Geometry check sheet. Reference: the model listing, model coordinates, mm. A direction names the side the tool comes from. Give positions to 0.01 mm unless a question says otherwise; leave off trailing zeros. Order: outer loops, then holes, each group sorted by start corner. A loop starts at its lowest first (then second) coordinate and runs counter-clockwise, first axis right, second up. Notation, with made-up numbers: M -8.75,83.25 L 16.25,83.25 A37 cw 16.25,119.25 Z; hole C 40.5,72.5 d1. An arc over 180 degrees is marked long. Answer as CSV lines item,"result". Start each with the question number.
Q1. Thickness scan on line 1 (Y direction, x = 0, z = -1.7); line 2 (X direction, y = -3.25, z = -8.25); line 3 (Y direction, x = 0, z = -4.45). Record the ranges inside material, lowest first.
Q2. Section check A-A, the plane x = 0. Record the boundary of the cut face in (y, z).
Q3. Section check D-D, the plane z = -1.75. Record the boundary of the cut face in (x, y), then the cut area to 3 significant figures.
Q4. Set-up check for faces 1 (the conical face through (-0.486, -2.187, -12.464)), 2 (the cylindrical face through (-1.886, -8.493, -2.282)), 3 (the cylindrical face through (-3.03, -13.67, -2.06)): record each of +Z, -Z, +X, -X, +Y, -Y from which the full face is reachable in a straight line by a thin tool's end or side.
Q5. Go/stop test with flat-tipped pins: pin 1 (4 mm diameter, centred on x = -6.5, y = -3, fed in from -Z); pin 2 (1.5 mm diameter, centred on x = -5.5, z = -9, fed in from +Y); pin 3 (1 mm diameter, centred on y = 10.5, z = -1.5, fed in from -X). Record where each tip stops, or that it passes through.
Q6. Section check B-B, the plane z = -5.25. Record the boundary of the cut face in (x, y).
Q7. Mould release check, pull along Z, two halves, no side actions. Record for faces 4 (the cylindrical face through (6.691, -12.864, -0.659)), 5 (the conical face through (-0.29, -1.29, -8.57)), 6 (the flat face through (-3, -9.5, 0)): +Z half, -Z half, draft (parallel to the pull), parting line (faces both ways), or undercut.
```python
from build123d import *


with BuildPart() as part:
    # 草图1 → 旋转1 (revolve)
    with BuildSketch(Plane(origin=(0, 0, 0), x_dir=(1, 0, 0), z_dir=(0, 1, 0))):
        with BuildLine():
            Line((0, 12.802374441), (0, 8.802374441))
            ThreePointArc((0, 8.802374441), (0.35150636, 8.781710488), (0.698170379, 8.720003294))
            Line((0.698170379, 8.720003294), (10.7, 6.326627875))
            Line((10.7, 6.326627875), (10.7, 3.6))
            Line((10.7, 3.6), (8.7, 3.6))
            Line((8.7, 3.6), (8.7, 1))
            Line((8.7, 1), (9.7, 0))
            Line((9.7, 0), (14.5, 0))
            Line((14.5, 0), (14.5, 1.300002326))
            Line((14.5, 1.300002326), (14.000000007, 1.300002326))
            Line((14.000000007, 1.300002326), (14.000000007, 2.800002326))
            ThreePointArc((14.000000007, 2.800002326), (14.955727499, 3.755729817), (14.000000007, 4.711457309))
            Line((14.000000007, 4.711457309), (14.000000007, 7.711454982))
            ThreePointArc((14.000000007, 7.711454982), (14.948966073, 8.553699236), (14.225360777, 9.595959929))
            Line((14.225360777, 9.595959929), (1.629064218, 12.610175098))
            ThreePointArc((1.629064218, 12.610175098), (0.820181506, 12.75415855), (0, 12.802374441))
        make_face()
    revolve(axis=Axis((0, 0, -12.802374441), (0, 0, 1)))


solid = part.part
```
Answer block:
1,line 1,"y = -14 to -8.7, 8.7 to 14"
1,line 2,"x = -14.5 to 14.5"
1,line 3,"y = -14.66 to -10.7, 10.7 to 14.66"
2,outline,"M -14.5,-1.3 L -14,-1.3 L -14,-2.8 A0.96 ccw -14,-4.71 L -14,-7.71 A0.96 ccw -14.23,-9.6 L -1.63,-12.61 A7 ccw 1.63,-12.61 L 14.23,-9.6 A0.96 ccw 14,-7.71 L 14,-4.71 A0.96 ccw 14,-2.8 L 14,-1.3 L 14.5,-1.3 L 14.5,0 L 9.7,0 L 8.7,-1 L 8.7,-3.6 L 10.7,-3.6 L 10.7,-6.33 L 0.7,-8.72 A3 cw -0.7,-8.72 L -10.7,-6.33 L -10.7,-3.6 L -8.7,-3.6 L -8.7,-1 L -9.7,0 L -14.5,0 Z"
3,outline,"C 0,0 d28; hole C 0,0 d17.4"
3,area,"378 mm2"
4,face 1,"-Z"
4,face 2,"+Z"
4,face 3,"none"
5,pin 1,"stops at z = -11.77"
5,pin 2,"stops at y = 14.16"
5,pin 3,"stops at x = -10.46"
6,outline,"C 0,0 d28; hole C 0,0 d21.4"
7,face 4,"draft"
7,face 5,"undercut"
7,face 6,"+Z half"
